Read the model definition and answer for the solid it produces. Units are mm, in the model's axes. A direction names the side the tool comes from. Give positions to 0.01 mm unless a question says otherwise; leave off trailing zeros. Write each loop counter-clockwise with the first axis right and the second up, starting at its lowest first coordinate (ties: lowest second). Pieces come first, ordered by that corner, then holes. Notation, with made-up numbers: (80, 68) -> (131, 68) arc R33 ccw to (131, 103) -> close; hole circle Ø2 at (80, 45). An arc over 180 degrees is marked (long way). Use a Markdown table: item, result.
Autodesk Inventor part; units mm, degrees
ref_plane "Work Plane1" through (-1, 0, 0) normal (0, 0, 1) x (1, 0, 0)
ref_plane "Work Plane4" through (-14.2, -9, 0.5) normal (-1, 0, 0) x (0, 0, 1)
ref_plane "Work Plane3" through (-10.8, -9.5, 0.5) normal (1, 0, 0) x (0, 0, -1)
ref_plane "Work Plane1" through (-1, 0, 0) normal (0, 0, 1) x (1, 0, 0)
sketch "Sketch1" plane through (-1, 0, 0) normal (0, 0, 1) x (1, 0, 0)
  line L0 (-7, 0) -> (-5, 0)
  line L1 (-5, 0) -> (-5, 0.5)
  line L2 (-5, 0.5) -> (-7, 0.5)
  line L3 (-7, 0.5) -> (-7, 0)
  line L4 (-5, 0) -> (-5, -0.4)
  line L5 (-7, 0) -> (-7, -0.4)
  line L6 (-1, 0) -> (-1, -0.4)
  line L7 (1, 0) -> (1, -0.4)
  line L8 (1, -8.6) -> (1, -9)
  line L9 (-1, -8.6) -> (-1, -9)
  line L10 (-5, -8.6) -> (-5, -9)
  line L11 (-7, -8.6) -> (-7, -9)
  line L12 (-7, -9.5) -> (-5, -9.5)
  line L13 (-5, -9.5) -> (-5, -9)
  line L14 (-5, -9) -> (-7, -9)
  line L15 (-7, -9) -> (-7, -9.5)
  line L16 (-1, -9.5) -> (1, -9.5)
  line L17 (1, -9.5) -> (1, -9)
  line L18 (1, -9) -> (-1, -9)
  line L19 (-1, -9) -> (-1, -9.5)
  line L20 (-1, 0) -> (1, 0)
  line L21 (1, 0) -> (1, 0.5)
  line L22 (1, 0.5) -> (-1, 0.5)
  line L23 (-1, 0.5) -> (-1, 0)
  line L24 (2.4038, -9) -> (-10, -9)
  line L25 (2.4038, 0) -> (-10, 0)
  line L26 (-13.2, -9) -> (2.9, -9)
  line L27 (2.9, -9) -> (2.9, 0)
  line L28 (2.9, 0) -> (-13.2, 0)
  line L29 (-13.2, 0) -> (-13.2, -9)
  line L30 (2.7, -2.7) -> (2.7, -1.9958)
  line L31 (-13, -9) -> (-13, -5.4522)
  point P0 (0.7, -9)
  point P1 (1, 0)
  point P2 (-1, 0)
  point P3 (-5, 0)
  point P4 (-7, 0)
  point P5 (1, 0)
  dimension "d89" = 0.5
  dimension "d90" = 0.2
  dimension "d125" = 0.2
extrude "main" add sketch "Sketch1" along normal blind 0.5
sketch "Sketch2" plane through (-1, 0, 0) normal (0, 0, -1) x (-1, 0, 0)
  line L0 (13, 0) -> (-2.4038, 0)
  line L1 (-2.4038, -9) -> (13, -9)
  line L2 (7, 0.5) -> (7, 0)
  line L3 (5, 0) -> (5, 0.5)
  line L4 (-1, 0) -> (-1, 0.5)
  line L5 (1, 0.5) -> (-1, 0.5)
  line L6 (-1, 0.5) -> (-1, 0.1)
  line L7 (-1, 0.1) -> (1, 0.1)
  line L8 (1, 0.1) -> (1, 0.5)
  line L9 (7, -9) -> (7, -9.5)
  line L10 (7, -9.5) -> (5, -9.5)
  line L11 (5, -9.5) -> (5, -9.1)
  line L12 (5, -9.1) -> (7, -9.1)
  line L13 (7, -9.1) -> (7, -9.5)
  line L14 (-1, -9.5) -> (-1, -9)
  line L15 (1, -9) -> (1, -9.5)
  line L16 (-1, -9.5) -> (1, -9.5)
  line L17 (1, -9.5) -> (1, -9.1)
  line L18 (1, -9.1) -> (-1, -9.1)
  line L19 (-1, -9.1) -> (-1, -9.5)
  line L20 (5, 0.5) -> (7, 0.5)
  line L21 (7, 0.5) -> (5, 0.5)
  line L22 (5, 0.5) -> (5, 0.1)
  line L23 (5, 0.1) -> (7, 0.1)
  line L24 (7, 0.1) -> (7, 0.5)
  line L25 (1, 0.5) -> (1, 0)
  line L26 (-1, 0.5) -> (1, 0.5)
  point P0 (1, -9.5)
  point P1 (-1, -9.1)
  point P2 (-1, 0.5)
  dimension "d91" = 0.1
  dimension "d92" = 0.1
  dimension "d93" = 0.1
  dimension "d94" = 0.1
extrude "flaps" add sketch "Sketch2" along normal blind 2 contours L23 L3 L20 L2 | L7 L4 L5 L8 | L9 L10 L11 L12 | L18 L15 L16 L14
sketch "Sketch18" plane through (-1, 0, 0) normal (0, 0, -1) x (-1, 0, 0)
  line L0 (7, 0) -> (13.2, 0)
  line L1 (13.2, 0) -> (10.2, 0)
  line L2 (10.2, 0) -> (10.2, -0.4)
  line L3 (10.2, -0.4) -> (13.2, -0.4)
  line L4 (13.2, -0.4) -> (13.2, 0)
  line L5 (13.2, -9) -> (7, -9)
  line L6 (13.2, -9) -> (10.2, -9)
  line L7 (10.2, -9) -> (10.2, -8.6)
  line L8 (10.2, -8.6) -> (13.2, -8.6)
  line L9 (13.2, -8.6) -> (13.2, -9)
  line L10 (10, 0) -> (10, -0.4)
  line L11 (-1.3, -0.4) -> (10, -0.4)
  line L12 (-1.3, -8.6) -> (10, -8.6)
  point P0 (-1, 0)
  point P1 (10.2, 0)
  dimension "d95" = 0.2
extrude "Extrusion18" add sketch "Sketch18" along normal blind 2.4
ref_plane "Work Plane4" through (-14.2, -9, 0.5) normal (-1, 0, 0) x (0, 0, 1)
sketch "Sketch19" plane through (-14.2, -9, 0.5) normal (-1, 0, 0) x (0, 0, 1)
  line L0 (0, 9) -> (0, 0)
  line L1 (0, 9) -> (-3.9, 9)
  line L2 (-3.9, 9) -> (-3.9, 0)
  line L3 (-3.9, 0) -> (0, 0)
  line L4 (0, 0) -> (0, 9)
  line L5 (-3.9, 8.5) -> (-3.9, 0.5)
extrude "Extrusion19" add sketch "Sketch19" along normal blind 0.4
fillet "Fillet7" radius 0.3 4 edges at (-1, -9.5, 0.5) (-1, 0.5, 0.5) (-7, 0.5, 0.5) (-7, -9.5, 0.5)
fillet "Fillet9" radius 1.7 2 edges at (1.9, 0, 0.25) (1.9, -9, 0.25)
sketch "Sketch22" plane through (-8, -9.1, 0) normal (0, 1, 0) x (1, 0, 0)
  line L0 (0, 0.9) -> (2, 0.9)
  line L1 (0, 2.1) -> (0, 0.9)
  line L2 (2, 0.9) -> (2, 2.1)
  line L3 (6, 0.9) -> (8, 0.9)
  line L4 (8, 0.9) -> (8, 2.1)
  line L5 (6, 2.1) -> (8, 2.1)
  line L6 (6, 2.1) -> (6, 0.9)
  line L7 (2, 2.1) -> (0, 2.1)
  line L8 (0.1, 1.1) -> (1.9, 1.1)
  line L9 (1.9, 1.1) -> (1.9, 2)
  line L10 (1.9, 2) -> (0.1, 2)
  line L11 (0.1, 2) -> (0.1, 1.1)
  line L12 (6.1, 1.1) -> (7.9, 1.1)
  line L13 (7.9, 1.1) -> (7.9, 2)
  line L14 (7.9, 2) -> (6.1, 2)
  line L15 (6.1, 2) -> (6.1, 1.1)
  point P0 (8, 0)
  dimension "d134" = 0.1
  dimension "d135" = 0.2
  dimension "d136" = 0.1
  dimension "d137" = 0.1
  dimension "d138" = 0.1
  dimension "d139" = 0.1
  dimension "d140" = 0.1
extrude "Extrusion22" add sketch "Sketch22" along normal blind 0.3 contours L11 L10 L9 L8 | L15 L14 L13 L12
sketch "Sketch23" plane through (-2, 0.1, 0) normal (0, -1, 0) x (1, 0, 0)
  line L0 (1.9, -2) -> (0.1, -2)
  line L1 (0.1, -1.1) -> (1.9, -1.1)
  line L2 (0.1, -2) -> (0.1, -1.1)
  line L3 (1.9, -1.1) -> (1.9, -2)
  line L4 (-4.1, -1.1) -> (-4.1, -2)
  line L5 (-4.1, -2) -> (-5.9, -2)
  line L6 (-5.9, -1.1) -> (-4.1, -1.1)
  line L7 (-5.9, -2) -> (-5.9, -1.1)
  point P0 (2, 0)
extrude "Extrusion23" add sketch "Sketch23" along normal blind 0.3
chamfer "Chamfer6" distance 0.2 angle 45 4 edges at (-1, -8.8, -2) (-7, -8.8, -2) (-7, -0.2, -2) (-1, -0.2, -2)
fillet "Fillet11" radius 0.2 5 edges at (1.4021, -0.4979, 0.5) (1.4021, -8.5021, 0.5) (1.9, -4.5, 0.5) (-4, -9, 0.5) (-4, 0, 0.5)
sketch "Sketch9" plane through (-1, 0, 0.5) normal (0, 0, 1) x (1, 0, 0)
  line L0 (-15.2, -10) -> (-9.8, -10)
  line L1 (-9.8, -10) -> (-9.8, 1)
  line L2 (-9.8, 1) -> (-15.2, 1)
  line L3 (-15.2, 1) -> (-15.2, -10)
  line L4 (-13.2, 0) -> (-13.2, -9)
  line L5 (-13.2, -9) -> (-7, -9) construction
  line L6 (-7, -9) -> (-7, -10) construction
  line L7 (-7, 0.1) -> (-7, 0) construction
  line L8 (-7, 0) -> (-7, 1) construction
  point P0 (1, 0)
  dimension "d100" = 5.4
  dimension "d101" = 11
  dimension "d102" = 2
ref_plane "Work Plane3" through (-10.8, -9.5, 0.5) normal (1, 0, 0) x (0, 0, -1)
sketch "Sketch20" plane through (-10.8, -9.5, 0.5) normal (1, 0, 0) x (0, 0, -1)
  line L0 (-0.925, -0.1) -> (-0.275, -0.1)
  line L1 (-0.275, -0.1) -> (-0.275, 10.1)
  line L2 (-0.275, 10.1) -> (-0.925, 10.1)
  line L3 (-0.925, 10.1) -> (-0.925, -0.1)
  line L4 (0, -0.5) -> (-1.2, -0.5) construction
  line L5 (0, 10.5) -> (-1.2, 10.5) construction
  line L6 (-1.2, -0.5) -> (-1.2, 10.5) construction
  point P0 (0.5, 9.5)
  point P1 (0.4, -0.5)
  point P2 (0.4, 10.5)
  dimension "d105" = 0.275
  dimension "d106" = 0.65
  dimension "d107" = 0.4
  dimension "d108" = 0.4
sketch "Sketch24" plane through (-14.6, -9, 0.5) normal (-1, 0, 0) x (0, 0, 1)
  line L0 (-4.7023, 8.5) -> (-3.4, 8.5)
  line L1 (-3.4, 8.5) -> (-3.4, 0.5)
  line L2 (-3.4, 0.5) -> (-4.7023, 0.5)
  line L3 (-4.7023, 0.5) -> (-4.7023, 8.5)
  line L4 (0, 0) -> (0, 9)
  line L5 (0, 9) -> (-3.9, 9)
  line L6 (-3.9, 9) -> (-3.9, 0)
  line L7 (-3.9, 0) -> (0, 0)
  point P0 (-0.5, 9)
  point P1 (-4.0512, 8.5)
  dimension "d152" = 8
  dimension "d153" = 0.5
  dimension "d154" = 0.5
extrude "Extrusion24" cut sketch "Sketch24" against normal blind 10 contours L0 L6 L2 L3 | L0 L1 L2 L6
properties part number "np2alpha_cap_flex_top"
Item 1: A cutting plane is placed at D-D (x = -4). Give the vertices of the cut face in (y, z).
Return value:
| item | result |
|---|---|
| outline | (-9, 0) -> (0, 0) -> (0, 0.3) arc R0.2 ccw to (-0.2, 0.5) -> (-8.8, 0.5) arc R0.2 ccw to (-9, 0.3) -> close |
Item 2: For a pull along Y with two mould halves and no side action, classify faces 1 (the face through (-14.6, -4, -1)), 2 (the face through (-1, -9.5, -1)), 3 (the face through (-1, -9.1, -0.5)) as +Y half, -Y half, draft (parallel to the pull), parting line (faces both ways), or undercut.
Return value:
| item | result |
|---|---|
| face 1 | draft |
| face 2 | -Y half |
| face 3 | undercut |
Item 3: A tool of negligible diameter and unlimited length cuts with its end or side. For faces 4 (the face through (-13, -0.4, -1)), 5 (the face through (-13, -9, -1)), 6 (the face through (-13, 0, -1)), from which of +Z, -Z, +X, -X, +Y, -Y can it reach the whole face along a straight path? Write none if from no direction.
Return value:
| item | result |
|---|---|
| face 4 | -Z, +X |
| face 5 | +Z, -Z, -X, -Y |
| face 6 | +Z, -Z, -X, +Y |
Item 4: A cutting plane is placed at B-B (y = -7). Give the vertices of the cut face in (x, z), then the cut area to 3 significant figures.
Return value:
| item | result |
|---|---|
| outline | (-14.6, -2.9) -> (-14.2, -2.9) -> (-14.2, 0) -> (1.9, 0) -> (1.9, 0.3) arc R0.2 ccw to (1.7, 0.5) -> (-14.6, 0.5) -> close |
| area | 9.40 mm^2 |
Item 5: Straight lines are drawn through the part: line 1 along Y through (x, z) = (-12.25, -0.4); line 2 along Y through (x, z) = (-6.75, -1.75); line 3 along Z through (x, y) = (-8.75, -6.75). For each, find the intervals that lie inside material, in ascending order. Write a range as [from, to].
Return value:
| item | result |
|---|---|
| line 1 | [-9, -8.6], [-0.4, 0] |
| line 2 | [-9.5, -8.8], [-0.2, 0.5] |
| line 3 | [0, 0.5] |
Item 6: Each of these flat-tipped pins is pushed along its axis until it touches: P1, Ø2, axis at x = -9.5, y = -8.5, coming from the -Z side; P2, Ø1.7, axis at y = -5.5, z = -1.5, coming from the +X side; P3, Ø0.8, axis at y = -9, z = -1, coming from the +X side. Where does it stop, or does it pass through?
Return value:
| item | result |
|---|---|
| P1 | z = 0 |
| P2 | x = -14.2 |
| P3 | x = 0 |
Item 7: A cutting plane is placed at C-C (x = -13.5). Give the vertices of the cut face in (y, z), then the cut area to 3 significant figures.
Return value:
| item | result |
|---|---|
| outline | (-9, -2.4) -> (-8.6, -2.4) -> (-8.6, 0) -> (-0.4, 0) -> (-0.4, -2.4) -> (0, -2.4) -> (0, 0.5) -> (-9, 0.5) -> close |
| area | 6.42 mm^2 |
Item 8: A cutting plane is placed at A-A (z = -0.2). Give the vertices of the cut face in (x, y).
Return value:
| item | result |
|---|---|
| outline | (-14.6, -9) -> (-11.2, -9) -> (-11.2, -8.6) -> (-14.2, -8.6) -> (-14.2, -0.4) -> (-11.2, -0.4) -> (-11.2, 0) -> (-14.6, 0) -> close; (-8, -9.5) -> (-6, -9.5) -> (-6, -9.1) -> (-8, -9.1) -> close; (-8, 0.1) -> (-6, 0.1) -> (-6, 0.5) -> (-8, 0.5) -> close; (-2, -9.5) -> (0, -9.5) -> (0, -9.1) -> (-2, -9.1) -> close; (-2, 0.1) -> (0, 0.1) -> (0, 0.5) -> (-2, 0.5) -> close |
